```python
from build123d import *

# Parameters (mm, degrees)
F1_DEPTH    = 12
F3_T1_DEPTH = 27
F3_T3_DEPTH = 26.8975669154
F4_SIZE     = 1
F2_R        = 2.9
F5_DEPTH    = 12.001
F6_DEPTH    = 6


# Not quite as in the source:
# - a fillet or chamfer that OpenCascade refuses, or shapes differently, is made with other operations: its cross-section is extruded or revolved along the edge and cut away or added


with BuildPart() as f1:
    # F0 (on Top) → F1 (new body)
    with BuildSketch(Plane.XY):
        with BuildLine():
            Line((-24.8, 6), (-28, 6))
            Line((-28, 6), (-28, -6))
            Line((-28, -6), (28, -6))
            Line((28, -6), (28, -3.35))
            Line((28, -3.35), (22.7247340124, -3.35))
            ThreePointArc((22.7247340124, -3.35), (18, 0), (22.7247340124, 3.35))
            Line((22.7247340124, 3.35), (28, 3.35))
            Line((28, 3.35), (28, 6))
            Line((28, 6), (-18.1, 6))
            Line((-18.1, 6), (-18.1, 1.1747340124))
            ThreePointArc((-18.1, 1.1747340124), (-17.9503571611, 0.5958187644), (-17.9, 0))
            ThreePointArc((-17.9, 0), (-22.0458187644, -3.4996428389), (-24.8, 1.1747340124))
            Line((-24.8, 1.1747340124), (-24.8, 6))
        make_face()
    extrude(amount=F1_DEPTH)

    # F3: fillet of radius 3 on 5 edges, made by hand

    # F3_s2 → F3_t1 (cut)
    with BuildSketch(Plane.XY.offset(-7.5)):
        with BuildLine():
            ThreePointArc((-15.1, 6), (-17.2213203436, 5.1213203436), (-18.1, 3))
            Line((-18.1, 3), (-18.1, 6))
            Line((-18.1, 6), (-15.1, 6))
        make_face()
        with BuildLine():
            ThreePointArc((-27.8, 6), (-25.6786796564, 5.1213203436), (-24.8, 3))
            Line((-24.8, 3), (-24.8, 6))
            Line((-24.8, 6), (-27.8, 6))
        make_face()
        with BuildLine():
            ThreePointArc((-25, -6), (-27.1213203436, -5.1213203436), (-28, -3))
            Line((-28, -3), (-28, -6))
            Line((-28, -6), (-25, -6))
        make_face()
    extrude(amount=F3_T1_DEPTH, mode=Mode.SUBTRACT)

    # F3_s4 → F3_t3 (cut)
    with BuildSketch(Plane.XY.offset(-7.4487834577)):
        with BuildLine():
            ThreePointArc((25.0204866169, -3.35), (27.0142268206, -4.1083488229), (28, -6))
            Line((28, -6), (28, -3.35))
            Line((28, -3.35), (25.0204866169, -3.35))
        make_face()
        with BuildLine():
            ThreePointArc((28, 6), (27.0142268206, 4.1083488229), (25.0204866169, 3.35))
            Line((25.0204866169, 3.35), (28, 3.35))
            Line((28, 3.35), (28, 6))
        make_face()
    extrude(amount=F3_T3_DEPTH, mode=Mode.SUBTRACT)

    # F4
    f4_edges = [f1.edges().sort_by_distance(p)[0] for p in [
        (1.5, -6, 12),
        (1.5, -6, 0),
        (18, 0, 12),
        (-21.45, -3.55, 12),
        (18, 0, 0),
        (-21.45, -3.55, 0),
        (6.45, 6, 0),
        (6.45, 6, 12),
        (-18.1, 2.087367, 0),
        (-17.22132, 5.12132, 0),
        (-27.12132, -5.12132, 0),
        (-28, 1.5, 0),
        (-18.1, 2.087367, 12),
        (-17.22132, 5.12132, 12),
        (-27.12132, -5.12132, 12),
        (-28, 1.5, 12),
    ]]
    chamfer(f4_edges, length=F4_SIZE)

    # F2 (on face) → F5 (cut, through all)
    with BuildSketch(Plane(origin=(0, 6, 0), x_dir=(-1, 0, 0), z_dir=(0, 1, 0))):
        with Locations((-10.75, 6)):
            Circle(F2_R)
        with Locations((10.75, 6)):
            Circle(F2_R)
    extrude(amount=-F5_DEPTH, mode=Mode.SUBTRACT)

    # F2 (on face) → F6 (cut)
    with BuildSketch(Plane(origin=(0, 6, 0), x_dir=(-1, 0, 0), z_dir=(0, 1, 0))):
        Polygon((-7.8921161675, 10.95), (-13.6078838325, 10.95), (-16.465767665, 6), (-13.6078838325, 1.05), (-7.8921161675, 1.05), (-5.034232335, 6), align=None)
        with Locations((-10.75, 6)):
            Circle(F2_R, mode=Mode.SUBTRACT)
        Polygon((13.6078838325, 10.95), (7.8921161675, 10.95), (5.034232335, 6), (7.8921161675, 1.05), (13.6078838325, 1.05), (16.465767665, 6), align=None)
        with Locations((10.75, 6)):
            Circle(F2_R, mode=Mode.SUBTRACT)
    extrude(amount=-F6_DEPTH, mode=Mode.SUBTRACT)


solid = f1.part
```
The listing builds one solid part. Answer for the finished solid, in the listing's coordinates (mm). A direction names the side the tool comes from. Give positions to 0.01 mm unless a question says otherwise; leave off trailing zeros. Loops run counter-clockwise (first coordinate to the right, second up) from the corner with the lowest first, then second, coordinate; pieces in that order, holes last. Notation, with made-up numbers: (36.5, 32) - (89.5, 32) arc R10 ccw to (89.5, 39) - close; hole circle Ø11 at (19, 20). An arc over 180 degrees is marked (long way). Return JSON: item names as keys, results as strings. Group by question number.
1. Find section A-A (x = 21.55). Write down the section's boundary in (y, z), then the cut area to 3 significant figures.
2. Which of the six approach directions +Z, -Z, +X, -X, +Y, -Y give full straight-line access (tool end or side, diameter ignored) to faces 4 (the flat face through (-17.6, 2.1, 11.5)), 5 (the flat face through (-17.6, 2.1, 0.5)), 6 (the flat face through (-13.2, 0, 8.3)), 7 (the cylindrical face through (-7.853, -2.958, 6.128)), 8 (the cylindrical face through (18, 0, 6))?
3. Find section D-D (x = -21.45). Write down the section's boundary in (y, z).
4. Straight lines are drawn through the part: line 1 (Y direction, x = 23, z = 3.25); line 2 (Z direction, x = 10.75, y = -1.8); line 3 (X direction, y = -5.5, z = 4.5). For each, find the intervals that lie inside material, in ascending order. Write a range as [from, to].
5. Find section C-C (x = 10.75). Write down the section's boundary in (y, z), then the cut area to 3 significant figures.
6. Find section B-B (z = 5.5). State how many separate pieces and enclosed holes the cut face has, then the cut area to 3 significant figures.
7. Given pin 1 Ø5 at (x, z) = (-8, 8) entering from +Y; pin 2 Ø6 at (y, z) = (-1.5, 9.5) entering from +X, each flat-ended and moving along its own axis, determine where each tip first touches the part or whether it passes through.
8. Determine the mould class of faces 1 (the conical face through (-26.71, -4.68, 0.4)), 2 (the flat face through (-6.483, 3.042, 8.51)), 3 (the flat face through (24, 3.35, 6)) for opening direction Z: pulls with the +Z half, pulls with the -Z half, needs draft (parallel to the pull), parting line crosses it, or undercut.
Verdict:
{
 "1": {"outline": "(-6, 1) - (-5, 0) - (-4.55, 0) - (-3.55, 1) - (-3.55, 11) - (-4.55, 12) - (-5, 12) - (-6, 11) - close; (3.55, 1) - (4.55, 0) - (5, 0) - (6, 1) - (6, 11) - (5, 12) - (4.55, 12) - (3.55, 11) - close", "area": "54.8 mm^2"},
 "2": {"face 4": "+Z, +Y", "face 5": "-Z, +Y", "face 6": "+Y", "face 7": "+Y, -Y", "face 8": "+Z, -Z"},
 "3": {"outline": "(-6, 1) - (-5, 0) - (-4.55, 0) - (-3.55, 1) - (-3.55, 11) - (-4.55, 12) - (-5, 12) - (-6, 11) - close"},
 "4": {"line 1": "y = [-6, -3.35], [3.35, 6]", "line 2": "z = [0, 3.1], [8.9, 12]", "line 3": "x = [-26.66, -13.23], [-8.27, 8.27], [13.23, 27.9]"},
 "5": {"outline": "(-6, 1) - (-5, 0) - (5, 0) - (6, 1) - (6, 1.05) - (0, 1.05) - (0, 3.1) - (-6, 3.1) - close; (-6, 8.9) - (0, 8.9) - (0, 10.95) - (6, 10.95) - (6, 11) - (5, 12) - (-5, 12) - (-6, 11) - close", "area": "47.8 mm^2"},
 "6": {"separate pieces": "3", "enclosed holes": "0", "area": "340 mm^2"},
 "7": {"pin 1": "stops at y = 6", "pin 2": "stops at x = 27.38"},
 "8": {"face 1": "pulls with the -Z half", "face 2": "undercut", "face 3": "needs draft"}
}
